Here's how the part is built. I have some questions about the finished solid (model axes, mm). Coordinates: 2 decimals unless noted, no trailing zeros. Loops run counter-clockwise (first coordinate to the right, second up) from the corner with the lowest first, then second, coordinate; pieces in that order, holes last. Notation, with made-up numbers: (49.25, -24.75) - (90.25, -24.75) arc R8 ccw to (90.25, -15.75) - close; hole circle Ø5 at (24.5, -25). An arc over 180 degrees is marked (long way). Use a Markdown table: item, result.
Autodesk Inventor part; units mm, degrees
ref_plane "Work Plane1" through (0, 15, 0) normal (0, 1, 0) x (-1, 0, 0)
ref_plane "Work Plane2" through (0, -5, 0) normal (0, 1, 0) x (-1, 0, 0)
ref_plane "YZ Plane" through (0, 0, 0) normal (1, 0, 0) x (0, 1, 0)
sketch "Sketch1" plane through (0, 0, 0) normal (0, 1, 0) x (-1, 0, 0)
  circle A0 centre (0, 0) radius 15
  dimension "d0" = 30
ref_plane "Work Plane1" through (0, 15, 0) normal (0, 1, 0) x (-1, 0, 0)
sketch "Sketch2" plane through (0, 15, 0) normal (0, 1, 0) x (-1, 0, 0)
  circle A0 centre (0, 0) radius 6
  dimension "d2" = 12
loft "Loft1" add profiles "Sketch1", "Sketch2"
ref_plane "Work Plane2" through (0, -5, 0) normal (0, 1, 0) x (-1, 0, 0)
sketch "Sketch3" plane through (0, -5, 0) normal (0, 1, 0) x (-1, 0, 0)
  circle A0 centre (0, 0) radius 12.5
  dimension "d8" = 25
loft "Loft2" add profiles "Sketch3" section 1 edges at (15, 0, 0)
fillet "Fillet1" radius 2 3 edges at (15, 0, 0) (12.5, -5, 0) (6, 15, 0)
sketch "Sketch4" plane through (0, 15, 0) normal (0, 1, 0) x (1, 0, 0)
  point P0 (0, 0)
  point P1 (0, 0)
hole "Hole1" at (0, 15, 0) direction (0, -1, 0) diameter 8 depth 15 tip angle 118
thread "Thread1"
properties part number "Foot"
Q1. I want a section at B-B, the plane y = -3.5. Write out the boundary of the cut face in (x, z).
Check values:
| item | result |
|---|---|
| outline | circle Ø26.5 at (0, 0) |
Q2. Please list where these lines run through material, in increasing order: L1, parallel to X at y = 11.25, z = 0; L2, parallel to X at y = 9, z = 0; L3, parallel to Z at x = 0, y = 7. Write a range as from..to.
Check values:
| item | result |
|---|---|
| L1 | -8.25..-4, 4..8.25 |
| L2 | -9.6..-4, 4..9.6 |
| L3 | -10.8..-4, 4..10.8 |
Q3. If we mould it in two halves opening along X, with no side actions, what happens to faces 1 (the face through (4, 15, 2)), 2 (the face through (-7.579, 11.756, -2.387)), 3 (the face through (3.905, 7.395, -0.867))? For each: pulls with the +X half, pulls with the -X half, needs draft (parallel to the pull), parting line crosses it, or undercut.
Check values:
| item | result |
|---|---|
| face 1 | needs draft |
| face 2 | parting line crosses it |
| face 3 | undercut |
Q4. Will these pins go through, and if not, where does the flat tip stop? P1, Ø12, axis at x = -4, y = 12, coming from the -Z side; P2, Ø4, axis at y = 11, z = -3.5, coming from the -X side; P3, Ø6, axis at y = 2, z = 5.5, coming from the -X side.
Check values:
| item | result |
|---|---|
| P1 | z = -11.02 |
| P2 | x = -9.11 |
| P3 | x = -14.37 |
Q5. I want a section at A-A, the plane y = 6.5. Write out the boundary of the cut face in (x, z), then the cut area to 3 significant figures.
Check values:
| item | result |
|---|---|
| outline | circle Ø22.2 at (0, 0); hole circle Ø8 at (0, 0) |
| area | 337 mm^2 |
